from build123d import *

# Parameters (mm, degrees)
SKETCH1_R                                       = 3.5
BOSS_EXTRUDE1_DEPTH                             = 16.5
CHAMFER1_SIZE                                   = 0.5
SKETCH2_R                                       = 3
BOSS_EXTRUDE2_DEPTH                             = 10.5
CSK_FOR_M4_FLAT_HEAD_MACHINE_SCREW1_D           = 4.2
CSK_FOR_M4_FLAT_HEAD_MACHINE_SCREW1_CSINK_D     = 5.5
CSK_FOR_M4_FLAT_HEAD_MACHINE_SCREW1_CSINK_ANGLE = 90


with BuildPart() as part:
    # Sketch1 → Boss-Extrude1 (new body)
    with BuildSketch(Plane.XY):
        Circle(SKETCH1_R)
    extrude(amount=BOSS_EXTRUDE1_DEPTH)

    # Chamfer1
    chamfer1_edges = [part.edges().sort_by_distance(p)[0] for p in [
        (-3.5, 0, 16.5),
    ]]
    chamfer(chamfer1_edges, length=CHAMFER1_SIZE)

    # Sketch2 → Boss-Extrude2 (add)
    with BuildSketch(Plane.XY.offset(16.5)):
        with Locations(Location((0, 0, 0), (0, 0, 180))):
            Circle(SKETCH2_R)
    extrude(amount=BOSS_EXTRUDE2_DEPTH)

    # CSK for M4 Flat Head Machine Screw1 (through all)
    with Locations(Plane(origin=(0, 0, 0), x_dir=(-1, 0, 0), z_dir=(0, 0, -1))):
        with Locations((0, 0)):
            CounterSinkHole(CSK_FOR_M4_FLAT_HEAD_MACHINE_SCREW1_D / 2, CSK_FOR_M4_FLAT_HEAD_MACHINE_SCREW1_CSINK_D / 2, counter_sink_angle=CSK_FOR_M4_FLAT_HEAD_MACHINE_SCREW1_CSINK_ANGLE)


solid = part.part
Build history of the part. All positions in model axes, mm. Round coordinates to 2 decimals unless told otherwise and drop trailing zeros. Loops run counter-clockwise (first coordinate to the right, second up) from the corner with the lowest first, then second, coordinate; pieces in that order, holes last. Notation, with made-up numbers: (31.25, -14) -> (35.25, -14) arc R35 ccw to (35.25, 18) -> close; hole circle Ø5 at (49, 11). An arc over 180 degrees is marked (long way). Use CSV: the item, a comma, the result in double quotes. Start each with the question number.
Q1. Saw through at C-C on z = 13.25. Give the cut face in (x, y).
Q2. Mould opens along Y. For faces 1 (the face through (-2.86, -0.9, 21.68)), 2 (the face through (2.003, 0.631, 14.009)), 3 (the face through (-3, -1, 0)) say: +Y half, -Y half, draft (parallel to the pull), parting line (faces both ways), or undercut.
Q3. Saw through at D-D on z = 17.75. Give the cut face in (x, y), and give its area (3 significant figures).
Q4. Drill centre lines: L1, parallel to Y at x = 0, z = 13.5; L2, parallel to Y at x = -0.5, z = 3.75. Where is each one in solid material? Low to high.
Q5. Flat gauge pins, fed straight in: pin 1 Ø4 at (x, y) = (0, 0) entering from -Z; pin 2 Ø2 at (x, z) = (2.5, 15) entering from -Y; pin 3 Ø1 at (y, z) = (1, 7) entering from -X. Where does each tip first touch, or does it go through?
Q6. Saw through at A-A on x = 0. Give the cut face in (y, z).
Solutions:
1,outline,"circle Ø7 at (0, 0); hole circle Ø4.2 at (0, 0)"
2,face 1,"parting line"
2,face 2,"undercut"
2,face 3,"draft"
3,outline,"circle Ø6 at (0, 0); hole circle Ø4.2 at (0, 0)"
3,area,"14.4 mm^2"
4,L1,"y = -3.5 to -2.1, 2.1 to 3.5"
4,L2,"y = -3.46 to -2.04, 2.04 to 3.46"
5,pin 1,"passes through"
5,pin 2,"stops at y = -3.16"
5,pin 3,"stops at x = -3.46"
6,outline,"(-3.5, 0) -> (-2.75, 0) -> (-2.1, 0.65) -> (-2.1, 27) -> (-3, 27) -> (-3, 16.5) -> (-3.5, 16) -> close; (2.1, 0.65) -> (2.75, 0) -> (3.5, 0) -> (3.5, 16) -> (3, 16.5) -> (3, 27) -> (2.1, 27) -> close"
